Source: CAD feature listing. Evaluate the final solid. Frame: model axes, mm. A direction names the side the tool comes from. Coordinates: 2 decimals unless noted, no trailing zeros. Loops run counter-clockwise (first coordinate to the right, second up) from the corner with the lowest first, then second, coordinate; pieces in that order, holes last.
Item 1: Pin query (flat end, axial travel): pin 1 Ø10 at (x, y) = (24, -11.5) entering from +Z; pin 2 Ø0.6 at (x, y) = (-33.5, 21) entering from +Z; pin 3 Ø10 at (y, z) = (-10, -8) entering from +X. Return the tip coordinate at first contact, or that it passes through.
Item 2: Reachability of faces 1 (the cylindrical face through (0.71, 18.9, -31.93)), 2 (the cylindrical face through (-0.1, -20.5, 17.5)), 3 (the flat face through (12, -21.5, 1)), 4 (the flat face through (-35, -20, 30)), 5 (the cylindrical face through (0.714, -20.297, -33.359)) from +Z, -Z, +X, -X, +Y, -Y: full face, straight path, thin tool, end or side. Return the list, or none.
Item 3: Line query: probe 1 along Y at (x, z) = (-41.5, 10.5); probe 2 along Z at (x, y) = (-16.5, 2); probe 3 along Y at (x, z) = (1.5, 3.5). Output: solid intervals per line, ascending.
Item 4: Pull-direction query (Z, two-part tool) for faces 6 (the cylindrical face through (0.1, -20.5, -19.5)), 7 (the cylindrical face through (0.714, 20.359, -33.297)), 8 (the flat face through (30, -20, 30)); classes: +Z half, -Z half, draft (parallel to the pull), parting line (faces both ways), or undercut.
Item 5: Section query B-B, the plane z = 19. Return the cut outline in (x, y), then the cut area to 3 significant figures.
Item 6: Section query C-C, the plane y = -8. Return the cut outline in (x, z).
Item 7: Section query A-A, the plane x = 0. Return the cut outline in (y, z).
```python
from build123d import *

# Parameters (mm, degrees)
SM_BASE_FLANGE_1_DEPTH = 51
CUT_EXTRUDE_1_REACH    = 77.102
SKETCH_3_W             = 5
SKETCH_3_H             = 10
CUT_EXTRUDE_2_DEPTH    = 76.101597853


# Sheet-metal steps are written as plain solids
with BuildPart() as part:
    # Sketch 1 → 基体-法兰1 (new, symmetric)
    with BuildSketch(Plane(origin=(0, 0, 0), x_dir=(0, 0, -1), z_dir=(1, 0, 0))):
        with BuildLine():
            Line((-32.5, -19.5), (30.5, -19.5))
            ThreePointArc((30.5, -19.5), (31.914213562, -18.914213562), (32.5, -17.5))
            Line((32.5, -17.5), (32.5, 17.5))
            ThreePointArc((32.5, 17.5), (31.914213562, 18.914213562), (30.5, 19.5))
            Line((30.5, 19.5), (-32.5, 19.5))
            Line((-32.5, 19.5), (-32.5, 21.5))
            Line((-32.5, 21.5), (30.5, 21.5))
            ThreePointArc((30.5, 21.5), (33.328427125, 20.328427125), (34.5, 17.5))
            Line((34.5, 17.5), (34.5, -17.5))
            ThreePointArc((34.5, -17.5), (33.328427125, -20.328427125), (30.5, -21.5))
            Line((30.5, -21.5), (-32.5, -21.5))
            Line((-32.5, -21.5), (-32.5, -19.5))
        make_face()
    extrude(amount=SM_BASE_FLANGE_1_DEPTH, both=True)

    # Sketch 2 → 切除-拉伸1 (cut, up to next)
    with BuildSketch(Plane.XZ.offset(21.5), mode=Mode.PRIVATE) as cut_extrude_1_sk1:
        with BuildLine():
            Line((5, 12.5), (5, -14.5))
            ThreePointArc((5, -14.5), (0, -19.5), (-5, -14.5))
            Line((-5, -14.5), (-5, 12.5))
            ThreePointArc((-5, 12.5), (0, 17.5), (5, 12.5))
        make_face()
    cut_extrude_1_tool1 = extrude(cut_extrude_1_sk1.sketch, amount=-CUT_EXTRUDE_1_REACH, mode=Mode.PRIVATE) & part.part
    add(cut_extrude_1_tool1.solids().sort_by_distance((0, -21.5, -1))[0], mode=Mode.SUBTRACT)

    # 草图3 → 切除-拉伸2 (cut, through all)
    with BuildSketch(Plane(origin=(0, 21.5, 0), x_dir=(1, 0, 0), z_dir=(0, 1, 0))):
        with Locations((-32.5, -32.5)):
            Rectangle(SKETCH_3_W, SKETCH_3_H)
        with Locations((32.5, -32.5)):
            Rectangle(SKETCH_3_W, SKETCH_3_H)
    extrude(amount=-CUT_EXTRUDE_2_DEPTH, mode=Mode.SUBTRACT)


solid = part.part
```
Verdict:
1. pin 1: stops at z = -32.5
1. pin 2: stops at z = 27.5
1. pin 3: passes through
2. face 1: +Z, +X, -X
2. face 2: -Y
2. face 3: +Z, -Z, +X, -X, -Y
2. face 4: +Z, +Y, -Y
2. face 5: -Z, +X, -X, -Y
3. probe 1: y = -21.5 to -19.5, 19.5 to 21.5
3. probe 2: z = -34.5 to -32.5
3. probe 3: y = 19.5 to 21.5
4. face 6: undercut
4. face 7: -Z half
4. face 8: draft
5. outline: (-51, -21.5) - (51, -21.5) - (51, -19.5) - (-51, -19.5) - close; (-51, 19.5) - (51, 19.5) - (51, 21.5) - (-51, 21.5) - close
5. area: 408 mm2
6. outline: (-51, -34.5) - (51, -34.5) - (51, -32.5) - (-51, -32.5) - close
7. outline: (-21.5, -30.5) arc R4 ccw to (-17.5, -34.5) - (17.5, -34.5) arc R4 ccw to (21.5, -30.5) - (21.5, 32.5) - (19.5, 32.5) - (19.5, -30.5) arc R2 cw to (17.5, -32.5) - (-17.5, -32.5) arc R2 cw to (-19.5, -30.5) - (-19.5, -19.5) - (-21.5, -19.5) - close; (-21.5, 17.5) - (-19.5, 17.5) - (-19.5, 32.5) - (-21.5, 32.5) - close
